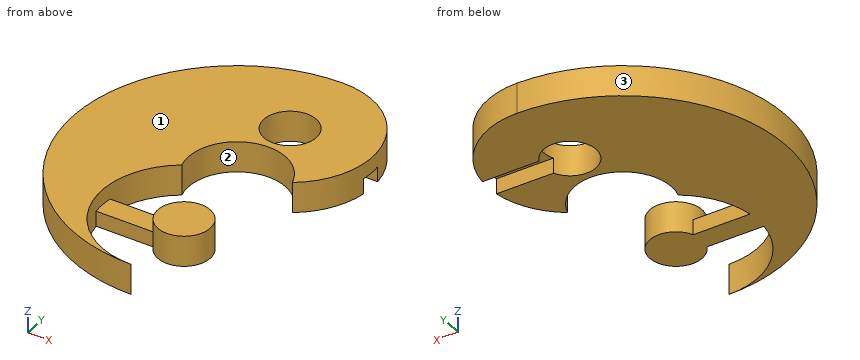
```python
from build123d import *

# Parameters (mm, degrees)
F0_R     = 6
F1_DEPTH = 7
F2_W     = 18.74953
F2_H     = 5
F3_DEPTH = 3.5
F4_W     = 22.433769
F4_H     = 5
F5_DEPTH = 3.5


with BuildPart() as f1:
    # F0 (on Top) → F1 (new body)
    with BuildSketch(Plane.XY):
        with BuildLine():
            ThreePointArc((10.602586, 3.2856), (17.909774, 24.3), (0, 37.5))
            ThreePointArc((0, 37.5), (-37.5, 0), (0, -37.5))
            ThreePointArc((0, -37.5), (-17.909774, -24.3), (-10.602586, -3.2856))
            ThreePointArc((-10.602586, -3.2856), (-3.2856, 10.602586), (10.602586, 3.2856))
        make_face()
        with Locations((0, 18.75)):
            Circle(F0_R, mode=Mode.SUBTRACT)
        with Locations((0, -18.75)):
            Circle(F0_R)
    extrude(amount=F1_DEPTH)

    # F2 (on Top) → F3 (join)
    with BuildSketch(Plane.XY):
        with Locations((-9.374765, -18.882733)):
            Rectangle(F2_W, F2_H)
    extrude(amount=F3_DEPTH)

    # F4 (on Top) → F5 (cut)
    with BuildSketch(Plane.XY):
        with Locations((11.216884, 18.75)):
            Rectangle(F4_W, F4_H)
    extrude(amount=F5_DEPTH, mode=Mode.SUBTRACT)


solid = f1.part
```
Build history of the part. All positions in model axes, mm. Face numbers are marked on the shaded views. Give positions to 0.01 mm unless a question says otherwise; leave off trailing zeros. Loops run counter-clockwise (first coordinate to the right, second up) from the corner with the lowest first, then second, coordinate; pieces in that order, holes last. Notation, with made-up numbers: (13.5, 44.5) - (63.5, 44.5) arc R31 ccw to (63.5, 77.5) - close; hole circle Ø2 at (12.25, 67). An arc over 180 degrees is marked (long way). Use a Markdown table: item, result.
(1) Band-saw the part on D-D (x = 7). Give the cut face in (y, z).
Taken from the geometry:
| item | result |
|---|---|
| outline | (8.61, 0) - (16.25, 0) - (16.25, 3.5) - (21.25, 3.5) - (21.25, 0) - (36.14, 0) - (36.14, 7) - (8.61, 7) - close |
(2) Wall check: line 1 along Y through (x, z) = (2.5, 4); line 2 along X through (y, z) = (17.5, 5); line 3 along X through (y, z) = (-23.5, 6.75). Give the ranges that are in metal, low to high.
Taken from the geometry:
| item | result |
|---|---|
| line 1 | -24.2 to -13.3, 10.81 to 13.3, 24.2 to 37.33 |
| line 2 | -33.17 to -5.87, 5.87 to 18.71 |
| line 3 | -29.22 to -18.14, -3.67 to 3.67 |
(3) Band-saw the part on B-B (z = 6). Give the cut face in (x, y).
Taken from the geometry:
| item | result |
|---|---|
| outline | (-10.6, -3.29) arc R11.1 cw to (10.6, 3.29) arc R18.75 ccw to (0, 37.5) arc R37.5 ccw to (0, -37.5) arc R18.75 cw to start; circle Ø12 at (0, -18.75); hole circle Ø12 at (0, 18.75) |
(4) Drop flat-ended pins along their axis: pin 1 Ø9.5 at (x, y) = (0, 18.75) entering from -Z; pin 2 Ø3 at (x, z) = (8.5, 5) entering from -Y; pin 3 Ø4 at (x, z) = (12, 1.5) entering from +Y; pin 4 Ø3 at (x, z) = (-8.5, 1) entering from +Y. Give the stop position or say it passes through.
Taken from the geometry:
| item | result |
|---|---|
| pin 1 | through |
| pin 2 | y = 4.82 |
| pin 3 | y = 34.61 |
| pin 4 | y = 36.84 |
(5) Band-saw the part on A-A (y = 18.75). Give the cut face in (x, z).
Taken from the geometry:
| item | result |
|---|---|
| outline | (-32.48, 0) - (-6, 0) - (-6, 7) - (-32.48, 7) - close; (6, 3.5) - (18.75, 3.5) - (18.75, 7) - (6, 7) - close |
(6) Pull direction Y, two halves, no side cores. Call the marked faces 1, 2 and 3: +Y half, -Y half, draft (parallel to the pull), parting line (faces both ways), or undercut.
Taken from the geometry:
| item | result |
|---|---|
| face 1 | draft |
| face 2 | undercut |
| face 3 | parting line |
